```python
from build123d import *

# Parameters (mm, degrees)
F1_DEPTH = 30
F2_R     = 5


with BuildPart() as f1:
    # F0 (on Top) → F1 (new body)
    with BuildSketch(Plane.XY):
        Polygon((50, 95.418446), (-50, -50), (50, -50), (50, -13.400296), (25, 0), (50, 11.463741), (50, 50), align=None)
    extrude(amount=F1_DEPTH)

    # F2
    f2_edges = [f1.edges().sort_by_distance(p)[0] for p in [
        (50, -50, 15),
        (-50, -50, 15),
    ]]
    fillet(f2_edges, radius=F2_R)


solid = f1.part
```
CAD build for the part. Positions are in the model's coordinates, mm. A direction names the side the tool comes from. Round coordinates to 2 decimals unless told otherwise and drop trailing zeros. Order: outer loops, then holes, each group sorted by start corner. A loop starts at its lowest first (then second) coordinate and runs counter-clockwise, first axis right, second up.
Q1. Wall check: L1, parallel to Y at x = 31.5, z = 26; L2, parallel to Y at x = 45.5, z = 23.25; L3, parallel to Y at x = 6.5, z = 22.5. Give the ranges that are in metal, low to high.
Q2. Two-plate mould, pull along Y, no slides. Class faces 3 (the flat face through (37.67, -6.79, 14.79)), 4 (the flat face through (50, -29, 15)), 5 (the cylindrical face through (48, -49, 15)): pulls with the +Y half, pulls with the -Y half, needs draft (parallel to the pull), parting line crosses it, or undercut.
Q3. Drop flat-ended pins along their axis: pin 1 (6 mm diameter, centred on x = 14, z = 17.5, fed in from +Y); pin 2 (5 mm diameter, centred on x = -22, z = 8.5, fed in from +Y); pin 3 (5 mm diameter, centred on x = 0, z = 10, fed in from +Y). Give the stop position or say it passes through.
Q4. Slice it at D-D (x = -22.5). Write the cut outline in (y, z).
Q5. Which spindle directions (+Z, -Z, +X, -X, +Y, -Y) get a long thin tool onto all of the face, cutting with end or side? Do faces 1 (the flat face through (37.325, 5.652, 14.79)), 2 (the flat face through (50, 53, 15)). Say none if no direction does.
Q6. Slice it at C-C (y = 4). Write the cut outline in (x, z), and give its area (3 significant figures).
Q7. Slice it at B-B (z = 4). Write the cut outline in (x, y).
Q8. Slice it at A-A (x = 33). Write the cut outline in (y, z).
Results below:
1. L1: y = -50 to -3.48, 2.98 to 68.52
1. L2: y = -49.97 to -10.99, 9.4 to 88.87
1. L3: y = -50 to 32.16
2. face 3: undercut
2. face 4: needs draft
2. face 5: pulls with the -Y half
3. pin 1: stops at y = 47.43
3. pin 2: stops at y = -5.65
3. pin 3: stops at y = 26.34
4. outline: (-50, 0) - (-10.01, 0) - (-10.01, 30) - (-50, 30) - close
5. face 1: +Z, -Z, +X
5. face 2: +Z, -Z, +X, +Y, -Y
6. outline: (-12.87, 0) - (33.72, 0) - (33.72, 30) - (-12.87, 30) - close
6. area: 1,400 mm2
7. outline: (-44.61, -42.17) arc R5 ccw to (-40.49, -50) - (45, -50) arc R5 ccw to (50, -45) - (50, -13.4) - (25, 0) - (50, 11.46) - (50, 95.42) - close
8. outline: (-50, 0) - (-4.29, 0) - (-4.29, 30) - (-50, 30) - close; (3.67, 0) - (70.7, 0) - (70.7, 30) - (3.67, 30) - close
